Geometry check sheet. Reference: the model listing, model coordinates, mm. Face numbers are marked on the shaded views. Give positions to 0.01 mm unless a question says otherwise; leave off trailing zeros. Write each loop counter-clockwise with the first axis right and the second up, starting at its lowest first coordinate (ties: lowest second). Pieces come first, ordered by that corner, then holes. Notation, with made-up numbers: (49.25, 84.5) - (90.25, 84.5) arc R25 ccw to (90.25, 105.5) - close; hole circle Ø8 at (36, -35.75). An arc over 180 degrees is marked (long way). One line per question, with ' | ' between items. Start each with the question number.
Q1. Section check A-A on y = 0. Record the boundary of the cut face in (x, z), and give its area (3 significant figures).
Q2. Section check C-C on z = 22. Record the boundary of the cut face in (x, y).
Q3. Release check for a two-part mould opening along Y. For the marked faces 1 and 2 record: +Y half, -Y half, draft (parallel to the pull), parting line (faces both ways), or undercut.
Q4. Gauge pin test, flat ends, axial feed: P1, Ø10, axis at x = 9, z = 14.5, coming from the +Y side; P2, Ø6, axis at y = 12, z = 12.5, coming from the -X side; P3, Ø3, axis at x = -14.5, z = 5.5, coming from the +Y side. Record the tip position at first contact, or that the pin passes through.
Q5. Thickness scan on L1, parallel to Y at x = 0, z = 8.5; L2, parallel to Y at x = 2, z = 23; L3, parallel to X at y = 9.5, z = 19.5. Record the ranges inside material, lowest first. Write a range as [from, to].
```python
from build123d import *

# Parameters (mm, degrees)
F0_R     = 25
F1_DEPTH = 25
F2_T     = -2.5
F3_R     = 22.5
F4_DEPTH = 2.5


with BuildPart() as f1:
    # F0 (on Top) → F1 (new body)
    with BuildSketch(Plane.XY):
        Circle(F0_R)
    extrude(amount=F1_DEPTH)

    # F2
    f2_openings = [f1.faces().sort_by_distance(p)[0] for p in [
        (0, 0, 25),
    ]]
    offset(amount=F2_T, openings=f2_openings)

    # F3 (on face) → F4 (cut)
    with BuildSketch(Plane.XY.offset(2.5)):
        Circle(F3_R)
    extrude(amount=-F4_DEPTH, mode=Mode.SUBTRACT)


solid = f1.part
```
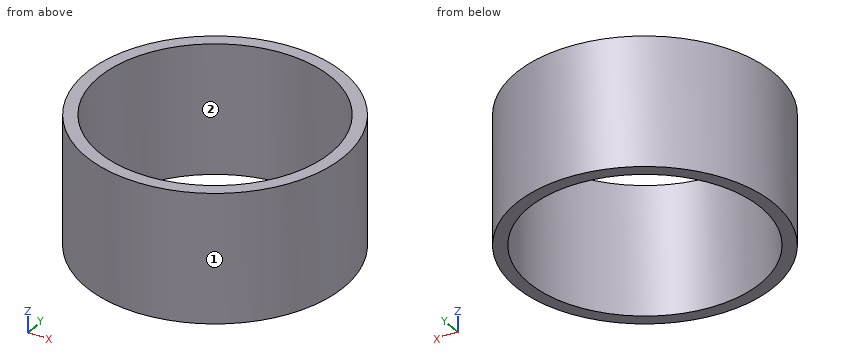
Working result:
1) outline: (-25, 0) - (-22.5, 0) - (-22.5, 25) - (-25, 25) - close; (22.5, 0) - (25, 0) - (25, 25) - (22.5, 25) - close | area: 125 mm2
2) outline: circle Ø50 at (0, 0); hole circle Ø45 at (0, 0)
3) face 1: parting line | face 2: undercut
4) P1: stops at y = 24.68 | P2: stops at x = -23.32 | P3: stops at y = 21.35
5) L1: y = [-25, -22.5], [22.5, 25] | L2: y = [-24.92, -22.41], [22.41, 24.92] | L3: x = [-23.12, -20.4], [20.4, 23.12]
